The figure shows three views and two pictorial views of one solid part (mm, origin at its lowest corner). Answer the questions. A direction names the side the tool comes from. Give positions to 0.01 mm unless a question says otherwise; leave off trailing zeros. Write each loop counter-clockwise with the first axis right and the second up, starting at its lowest first coordinate (ties: lowest second). Pieces come first, ordered by that corner, then holes. Notation, with made-up numbers: (-24, 47) -> (34, 47) arc R32 ccw to (34, 85) -> close; hole circle Ø10 at (-33.75, 19). An arc over 180 degrees is marked (long way). Use a Markdown table: item, result.
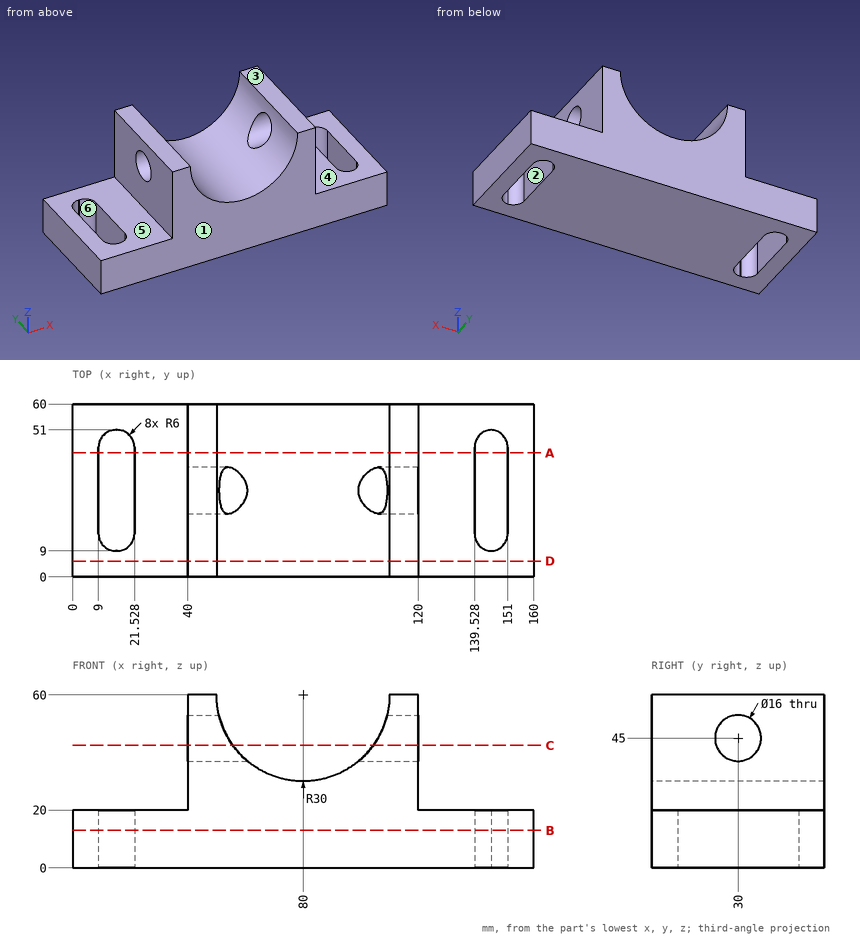
Item 1: A cutting plane is placed at C-C (z = 42.5). Give the vertices of the cut face in (x, y).
Return value:
| item | result |
|---|---|
| outline | (40, 0) -> (55.63, 0) -> (55.63, 22.4) -> (40, 22.4) -> close; (40, 37.6) -> (55.63, 37.6) -> (55.63, 60) -> (40, 60) -> close; (104.37, 0) -> (120, 0) -> (120, 22.4) -> (104.37, 22.4) -> close; (104.37, 37.6) -> (120, 37.6) -> (120, 60) -> (104.37, 60) -> close |
Item 2: A tool of negligible diameter and unlimited length cuts with its end or side. For the marked faces 4, 5 and 6, from which of +Z, -Z, +X, -X, +Y, -Y can it reach the whole face along a straight path? Write none if from no direction.
Return value:
| item | result |
|---|---|
| face 4 | +Z, +X, +Y, -Y |
| face 5 | +Z, -X, +Y, -Y |
| face 6 | +Z, -Z |
Item 3: A cutting plane is placed at B-B (z = 13). Give the vertices of the cut face in (x, y) (1 decimal), then the cut area to 3 significant figures.
Return value:
| item | result |
|---|---|
| outline | (0, 0) -> (160, 0) -> (160, 60) -> (0, 60) -> close; hole (9, 15) arc R6 ccw to (15, 9) -> (15.5, 9) arc R6 ccw to (21.5, 15) -> (21.5, 45) arc R6 ccw to (15.5, 51) -> (15, 51) arc R6 ccw to (9, 45) -> close; hole (139.5, 15) arc R6 ccw to (145.3, 9) arc R6 ccw to (151, 15) -> (151, 45) arc R6 ccw to (145.3, 51) arc R6 ccw to (139.5, 45) -> close |
| area | 8,650 mm^2 |
Item 4: Each of these flat-tipped pins is pushed along its axis until it touches: P1, Ø21, axis at y = 30, z = 45, coming from the +X side; P2, Ø12, axis at x = 29, y = 42, coming from the +Z side; P3, Ø18.5, axis at y = 30, z = 45, coming from the -X side. Where does it stop, or does it pass through?
Return value:
| item | result |
|---|---|
| P1 | x = 120 |
| P2 | z = 20 |
| P3 | x = 40 |
Item 5: A cutting plane is placed at A-A (y = 43). Give the vertices of the cut face in (x, z), then the cut area to 3 significant figures.
Return value:
| item | result |
|---|---|
| outline | (0, 0) -> (9, 0) -> (9, 20) -> (0, 20) -> close; (21.53, 0) -> (139.53, 0) -> (139.53, 20) -> (120, 20) -> (120, 60) -> (110, 60) arc R30 cw to (50, 60) -> (40, 60) -> (40, 20) -> (21.53, 20) -> close; (151, 0) -> (160, 0) -> (160, 20) -> (151, 20) -> close |
| area | 4,510 mm^2 |
Item 6: Straight lines are drawn through the part: line 1 along X through (y, z) = (38, 3); line 2 along Z through (x, y) = (49.75, 30); line 3 along Y through (x, z) = (111, 45). For each, find the intervals that lie inside material, in ascending order. Write a range as [from, to].
Return value:
| item | result |
|---|---|
| line 1 | [0, 9], [21.53, 139.53], [151, 160] |
| line 2 | [0, 37], [53, 60] |
| line 3 | [0, 22], [38, 60] |
Item 7: A cutting plane is placed at D-D (y = 5.5). Give the vertices of the cut face in (x, z).
Return value:
| item | result |
|---|---|
| outline | (0, 0) -> (160, 0) -> (160, 20) -> (120, 20) -> (120, 60) -> (110, 60) arc R30 cw to (50, 60) -> (40, 60) -> (40, 20) -> (0, 20) -> close |
Item 8: For a pull along Y with two mould halves and no side action, classify the marked faces 1, 2 and 3 as +Y half, -Y half, draft (parallel to the pull), parting line (faces both ways), or undercut.
Return value:
| item | result |
|---|---|
| face 1 | -Y half |
| face 2 | undercut |
| face 3 | draft |
